from build123d import *

# Parameters (mm, degrees)
SLITCUTSKE_W     = 5.336948004
SLITCUTSKE_H     = 0.71628
SLITCUT_DEPTH    = 6.860032
SLITCUTPAT_COUNT = 2
SLITCUTPAT_ANGLE = 90


with BuildPart() as part:
    # BodySke → Body (revolve)
    with BuildSketch(Plane.XY, mode=Mode.PRIVATE) as body_sk:
        Polygon((2.55778, 0.508), (2.55778, 0.889), (2.6924, 0.889), (2.6924, 3.043428), (2.02946, 3.706368), (2.02946, 5.78358), (2.3876, 6.14172), (2.3876, 6.858), (1.9812, 6.858), (2.17932, 8.6487), (2.17932, 9.00684), (1.88214, 10.4394), (0, 10.4394), (0, 0), (3.175, 0), (3.175, 0.508), align=None)
    revolve(body_sk.sketch.rotate(Axis((0, 0, 0), (0, 1, 0)), 90), axis=Axis((0, 0, 0), (0, 1, 0)))

    # SlitCutSke → SlitCut (cut)
    with BuildSketch(Plane(origin=(0, 10.4394, 0), x_dir=(-1, 0, 0), z_dir=(0, 1, 0))):
        Rectangle(SLITCUTSKE_W, SLITCUTSKE_H)
    slitcut = extrude(amount=-SLITCUT_DEPTH, mode=Mode.SUBTRACT)

    # SlitCutPat: SlitCut ×2 about axis
    slitcutpat_axis = Axis((0, 0, 0), (0, 1, 0))
    for i in range(1, SLITCUTPAT_COUNT):
        add(slitcut.rotate(slitcutpat_axis, i * SLITCUTPAT_ANGLE / (SLITCUTPAT_COUNT - 1)), mode=Mode.SUBTRACT)


solid = part.part
Geometry check sheet. Reference: the model listing, model coordinates, mm. A direction names the side the tool comes from. Round coordinates to 2 decimals unless told otherwise and drop trailing zeros. Loops run counter-clockwise (first coordinate to the right, second up) from the corner with the lowest first, then second, coordinate; pieces in that order, holes last. Notation, with made-up numbers: (33, 70.5) -> (72, 70.5) arc R10 cw to (72, 84.5) -> close; hole circle Ø5 at (18, -39.75). An arc over 180 degrees is marked (long way). Answer as a JSON object with one key per item and string values. Group by question number.
Item 1: Cross-section at C-C, the plane x = 0. Record the cut outline in (y, z) (3 decimals).
Item 2: Release check for a two-part mould opening along Y. For faces 4 (the face through (1, 10.439, 1)), 5 (the face through (1.45, 4.76, -1.42)), 6 (the face through (-1.459, 7.766, -1.485)), 7 (the face through (1.55, 8.83, -1.53)) record: pulls with the +Y half, pulls with the -Y half, needs draft (parallel to the pull), parting line crosses it, or undercut.
Item 3: Cross-section at D-D, the plane y = 2.25. Record the cut outline in (x, z).
Item 4: Cross-section at B-B, the plane z = 0. Record the cut outline in (x, y) (3 decimals).
Item 5: Thickness scan on line 1 along Y through (x, z) = (-2, -0.25); line 2 along X through (y, z) = (6.5, -2); line 3 along X through (y, z) = (9.5, -1). Record the ranges inside material, lowest first.
Item 6: Set-up check for faces 1 (the face through (-1.55, 8.83, 1.53)), 2 (the face through (-2.536, 0.701, 0.333)), 3 (the face through (-1, 6.858, 2)): record each of +Z, -Z, +X, -X, +Y, -Y from which the full face is reachable in a straight line by a thin tool's end or side.
Item 7: Depth check by flat-ended pin: pin 1 Ø2 at (x, y) = (1, 3) entering from -Z; pin 2 Ø1.5 at (y, z) = (3, -0.5) entering from -X; pin 3 Ø1.5 at (y, z) = (4, 2) entering from -X. Enter the tip coordinate at first touch or a pass-through.
Item 8: Cross-section at A-A, the plane y = 4.5. Record the cut outline in (x, z).
Determined:
{
 "1": {"outline": "(0, -3.175) -> (0.508, -3.175) -> (0.508, -2.558) -> (0.889, -2.558) -> (0.889, -2.692) -> (3.043, -2.692) -> (3.579, -2.156) -> (3.579, 2.156) -> (3.043, 2.692) -> (0.889, 2.692) -> (0.889, 2.558) -> (0.508, 2.558) -> (0.508, 3.175) -> (0, 3.175) -> close"},
 "2": {"face 4": "pulls with the +Y half", "face 5": "undercut", "face 6": "undercut", "face 7": "needs draft"},
 "3": {"outline": "circle Ø5.38 at (0, 0)"},
 "4": {"outline": "(-3.175, 0) -> (3.175, 0) -> (3.175, 0.508) -> (2.558, 0.508) -> (2.558, 0.889) -> (2.692, 0.889) -> (2.692, 3.043) -> (2.156, 3.579) -> (-2.156, 3.579) -> (-2.692, 3.043) -> (-2.692, 0.889) -> (-2.558, 0.889) -> (-2.558, 0.508) -> (-3.175, 0.508) -> close"},
 "5": {"line 1": "y = 0 to 3.58", "line 2": "x = -1.3 to -0.36, 0.36 to 1.3", "line 3": "x = -1.82 to -0.36, 0.36 to 1.82"},
 "6": {"face 1": "+Z, -X, +Y", "face 2": "none", "face 3": "+Z, -X"},
 "7": {"pin 1": "stops at z = -2.69", "pin 2": "stops at x = -2.69", "pin 3": "stops at x = -1.75"},
 "8": {"outline": "(-2, -0.36) arc R2.03 ccw to (-0.36, -2) -> (-0.36, -0.36) -> close; (-2, 0.36) -> (-0.36, 0.36) -> (-0.36, 2) arc R2.03 ccw to start; (0.36, -2) arc R2.03 ccw to (2, -0.36) -> (0.36, -0.36) -> close; (0.36, 0.36) -> (2, 0.36) arc R2.03 ccw to (0.36, 2) -> close"}
}
